from build123d import *

# Parameters (mm, degrees)
SKETCH_1_R      = 1.6
EXTRUDE_1_DEPTH = 5


with BuildPart() as part:
    # 草图1 → 凸台-拉伸1 (new body)
    with BuildSketch(Plane(origin=(0, 0, 0), x_dir=(1, 0, 0), z_dir=(0, 1, 0))):
        Polygon((-10, 35), (0, 35), (167, 35), (167, 65), (232, 65), (232, 15), (20, 15), (20, 0), (20, -35), (0, -35), (-10, -35), align=None)
        with Locations(Location((0, -20, 0), (0, 0, 270))):
            Circle(SKETCH_1_R, mode=Mode.SUBTRACT)
        with Locations(Location((0, 20, 0), (0, 0, 90))):
            Circle(SKETCH_1_R, mode=Mode.SUBTRACT)
        with Locations(Location((172, 29, 0), (0, 0, 270))):
            Circle(SKETCH_1_R, mode=Mode.SUBTRACT)
        with Locations(Location((172, 44, 0), (0, 0, 270))):
            Circle(SKETCH_1_R, mode=Mode.SUBTRACT)
        with Locations(Location((228, 29, 0), (0, 0, 270))):
            Circle(SKETCH_1_R, mode=Mode.SUBTRACT)
        with Locations(Location((228, 44, 0), (0, 0, 270))):
            Circle(SKETCH_1_R, mode=Mode.SUBTRACT)
    extrude(amount=EXTRUDE_1_DEPTH)


solid = part.part
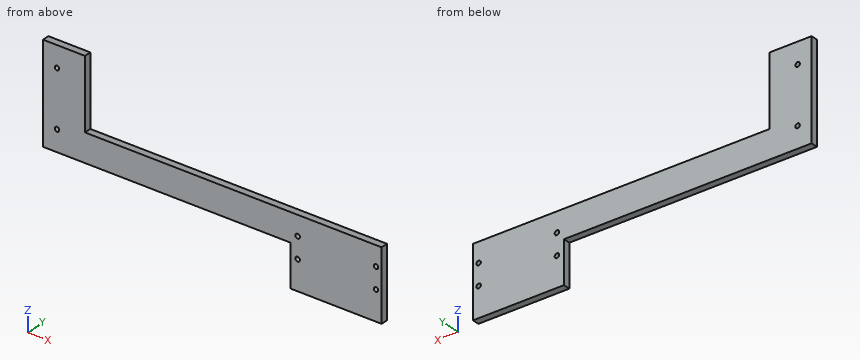
Model file for the job. Use its own axes, mm. Give positions to 0.01 mm unless a question says otherwise; leave off trailing zeros. Order: outer loops, then holes, each group sorted by start corner. A loop starts at its lowest first (then second) coordinate and runs counter-clockwise, first axis right, second up. Notation, with made-up numbers: (36, 6) -> (92, 6) arc R32 ccw to (92, 43) -> close; hole circle Ø1 at (19, 2.5). An arc over 180 degrees is marked (long way). Use CSV: the item, a comma, the result in double quotes.
1. Band-saw the part on B-B, the plane x = 25.5. Give the cut face in (y, z).
Outcome:
outline,"(0, -35) -> (5, -35) -> (5, -15) -> (0, -15) -> close"
2. Drill centre lines: line 1 along X through (y, z) = (2.6, -29); line 2 along X through (y, z) = (1.2, -44); line 3 along Z through (x, y) = (172, 3.45). Where is each one in solid material? Low to high. Write a range as from..to.
Outcome:
line 1,"-10..170.4, 173.6..226.4, 229.6..232"
line 2,"167..170.4, 173.6..226.4, 229.6..232"
line 3,"-65..-45.6, -42.4..-30.6, -27.4..-15"
3. Band-saw the part on A-A, the plane y = 2.9. Give the cut face in (x, z), then the cut area to 3 significant figures.
Outcome:
outline,"(-10, -35) -> (167, -35) -> (167, -65) -> (232, -65) -> (232, -15) -> (20, -15) -> (20, 35) -> (-10, 35) -> close; hole circle Ø3.2 at (0, -20); hole circle Ø3.2 at (0, 20); hole circle Ø3.2 at (172, -44); hole circle Ø3.2 at (172, -29); hole circle Ø3.2 at (228, -44); hole circle Ø3.2 at (228, -29)"
area,"8,240 mm²"
4. Band-saw the part on C-C, the plane z = 11.5. Give the cut face in (x, y).
Outcome:
outline,"(-10, 0) -> (20, 0) -> (20, 5) -> (-10, 5) -> close"
5. Drop flat-ended pins along their axis: pin 1 (1.5 mm diameter, centred on x = 147.5, y = 1.5, fed in from +Z); pin 2 (1 mm diameter, centred on y = 1.5, z = 5.5, fed in from +X). Give the stop position or say it passes through.
Outcome:
pin 1,"z = -15"
pin 2,"x = 20"
